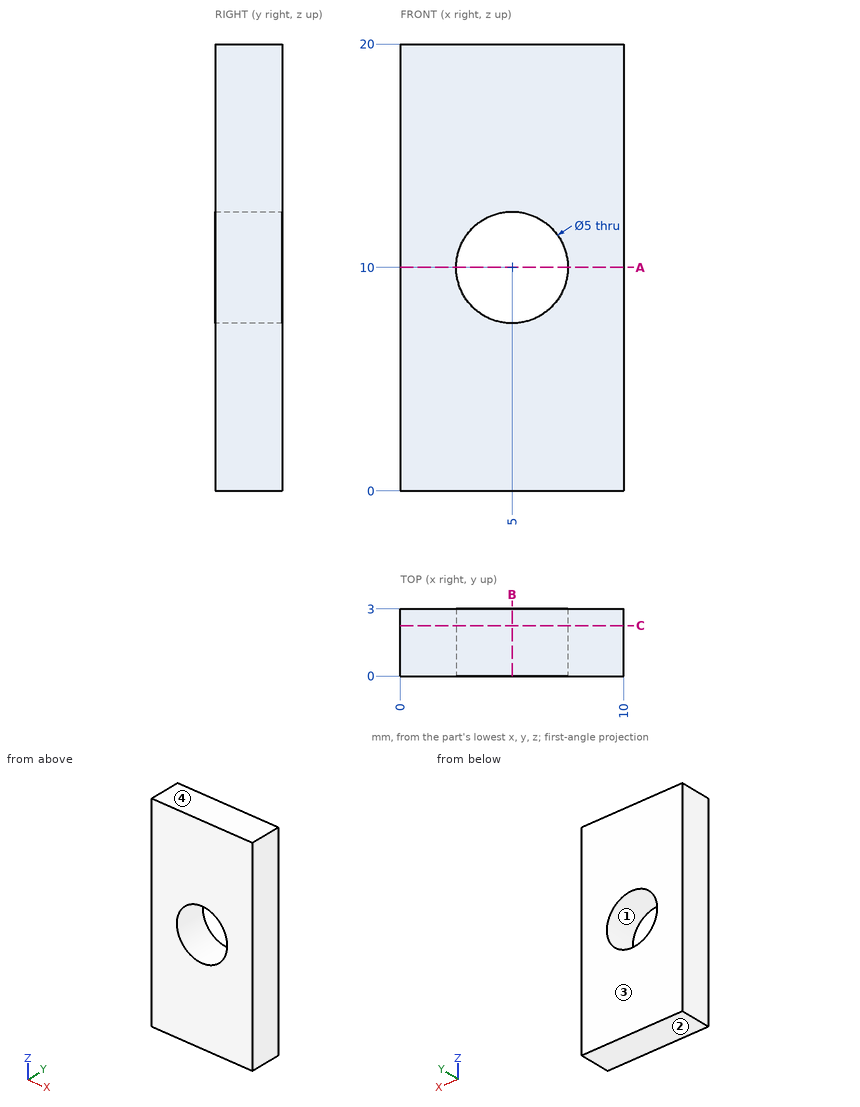
Verification items for this drawing (mm, ordinates from the low corner). Give positions to 0.01 mm unless a question says otherwise; leave off trailing zeros. Order: outer loops, then holes, each group sorted by start corner. A loop starts at its lowest first (then second) coordinate and runs counter-clockwise, first axis right, second up.
1) Cross-section at B-B (x = 5). Record the boundary of the cut face in (y, z).
Results are:
outline: (0, 0) - (3, 0) - (3, 7.5) - (0, 7.5) - close; (0, 12.5) - (3, 12.5) - (3, 20) - (0, 20) - close
2) Cross-section at A-A (z = 10). Record the boundary of the cut face in (x, y).
Results are:
outline: (0, 0) - (2.5, 0) - (2.5, 3) - (0, 3) - close; (7.5, 0) - (10, 0) - (10, 3) - (7.5, 3) - close
3) Material ranges on probe 1 along X at (y, z) = (1.5, 10); probe 2 along Z at (x, y) = (3.5, 1.7); probe 3 along Z at (x, y) = (3, 1.95), recorded low to high.
Results are:
probe 1: x = 0 to 2.5, 7.5 to 10
probe 2: z = 0 to 8, 12 to 20
probe 3: z = 0 to 8.5, 11.5 to 20
4) Cross-section at C-C (y = 2.25). Record the boundary of the cut face in (x, z), then the cut area to 3 significant figures.
Results are:
outline: (0, 0) - (10, 0) - (10, 20) - (0, 20) - close; hole circle Ø5 at (5, 10)
area: 180 mm2
5) Draft check along Z on the marked faces 1, 2, 3 and 4. Enter one of: released by +Z, released by -Z, zero draft, split by the parting line, or undercut.
Results are:
face 1: undercut
face 2: released by -Z
face 3: zero draft
face 4: released by +Z
